Answer from the drawing. Dimensions are ordinates in mm from the lowest x, y and z of the part. A direction names the side the tool comes from. Coordinates: 2 decimals unless noted, no trailing zeros. Order: outer loops, then holes, each group sorted by start corner. A loop starts at its lowest first (then second) coordinate and runs counter-clockwise, first axis right, second up. Notation, with made-up numbers: (54.25, 45.5) -> (86.25, 45.5) arc R19 ccw to (86.25, 59.5) -> close; hole circle Ø6 at (-37.5, 38.5). An arc over 180 degrees is marked (long way). Use CSV: the item, a comma, the result in double quotes.
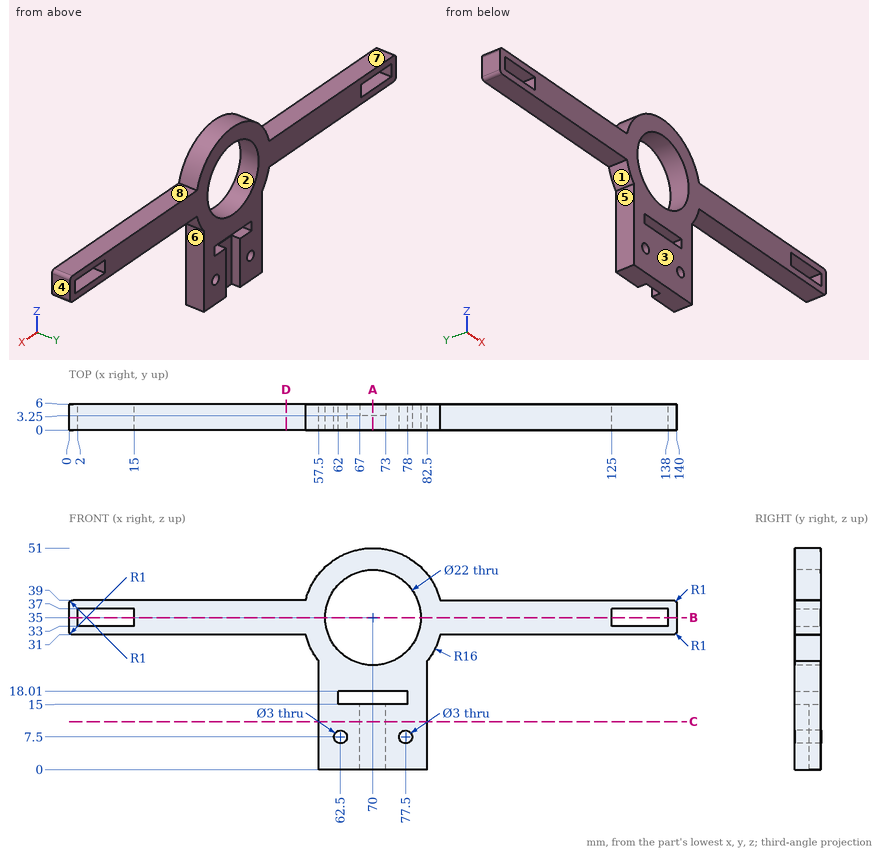
Item 1: Find section D-D, the plane x = 50. Give the vertices of the cut face in (y, z).
Return value:
outline,"(0, 31) -> (6, 31) -> (6, 39) -> (0, 39) -> close"
Item 2: A tool of negligible diameter and unlimited length cuts with its end or side. For the marked faces 5, 6, 7 and 8, from which of +Z, -Z, +X, -X, +Y, -Y can it reach the whole face along a straight path? Write none if from no direction.
Return value:
face 5,"-Z, -X, +Y, -Y"
face 6,"-Z, +X, +Y, -Y"
face 7,"+Z, -X, +Y, -Y"
face 8,"+Z, +X, +Y, -Y"
Item 3: The mould has two halves that part along X. Classify the marked faces 1, 2, 3 and 4: +X half, -X half, draft (parallel to the pull), parting line (faces both ways), or undercut.
Return value:
face 1,"-X half"
face 2,"undercut"
face 3,"draft"
face 4,"+X half"
Item 4: Find section B-B, the plane z = 35. Give the vertices of the cut face in (x, y).
Return value:
outline,"(0, 0) -> (2, 0) -> (2, 6) -> (0, 6) -> close; (15, 0) -> (59, 0) -> (59, 6) -> (15, 6) -> close; (81, 0) -> (125, 0) -> (125, 6) -> (81, 6) -> close; (138, 0) -> (140, 0) -> (140, 6) -> (138, 6) -> close"
Item 5: Find section A-A, the plane x = 70. Give the vertices of the cut face in (y, z), then the cut area to 3 significant figures.
Return value:
outline,"(0, 0) -> (3.25, 0) -> (3.25, 15) -> (0, 15) -> close; (0, 18.01) -> (6, 18.01) -> (6, 24) -> (0, 24) -> close; (0, 46) -> (6, 46) -> (6, 51) -> (0, 51) -> close"
area,"115 mm^2"
Item 6: Each of these flat-tipped pins is pushed along its axis until it touches: P1, Ø0.9, axis at y = 4, z = 16, coming from the -X side; P2, Ø3, axis at x = 10.5, y = 3, coming from the -Z side; P3, Ø5, axis at x = 70, z = 10, coming from the +Y side. Where does it stop, or does it pass through?
Return value:
P1,"stops at x = 57.5"
P2,"stops at z = 31"
P3,"stops at y = 3.25"
Item 7: Straight lines are drawn through the part: line 1 along X through (y, z) = (2, 7.5); line 2 along X through (y, z) = (4.75, 7.5); line 3 along Z through (x, y) = (13, 2.25). For each, find the intervals that lie inside material, in ascending order.
Return value:
line 1,"x = 57.5 to 61, 64 to 76, 79 to 82.5"
line 2,"x = 57.5 to 61, 64 to 67, 73 to 76, 79 to 82.5"
line 3,"z = 31 to 33, 37 to 39"
Item 8: Find section C-C, the plane z = 11. Give the vertices of the cut face in (x, y).
Return value:
outline,"(57.5, 0) -> (82.5, 0) -> (82.5, 6) -> (73, 6) -> (73, 3.25) -> (67, 3.25) -> (67, 6) -> (57.5, 6) -> close"
